Could you check a few things on this model? Use its own coordinates, in mm. Round coordinates to 2 decimals unless told otherwise and drop trailing zeros. Loops run counter-clockwise (first coordinate to the right, second up) from the corner with the lowest first, then second, coordinate; pieces in that order, holes last. Notation, with made-up numbers: M 49.5,-24.5 L 95.5,-24.5 A17 cw 95.5,8.5 Z; hole C 46.5,64 d7. An arc over 180 degrees is marked long. Answer in a Markdown table with one row per item.
```python
from build123d import *

# Parameters (mm, degrees)
ESQUISSE2_W             = 10
ESQUISSE2_H             = 10
BOSS_EXTRU_1_DEPTH      = 90
ESQUISSE3_W             = 10
ESQUISSE3_H             = 150
ESQUISSE3_R             = 2.5
BOSS_EXTRU_2_DEPTH      = 10
ESQUISSE4_R             = 2.5
ENL_V_MAT_EXTRU_1_DEPTH = 10
BOSS_EXTRU_3_DEPTH      = 10


with BuildPart() as part:
    # Esquisse2 → Boss.-Extru.1 (new body)
    with BuildSketch(Plane(origin=(0, 0, 0), x_dir=(0, 0, -1), z_dir=(1, 0, 0))):
        Rectangle(ESQUISSE2_W, ESQUISSE2_H)
    extrude(amount=BOSS_EXTRU_1_DEPTH)

    # Esquisse3 → Boss.-Extru.2 (add)
    with BuildSketch(Plane(origin=(90, 0, 0), x_dir=(0, 0, -1), z_dir=(1, 0, 0))):
        with Locations((0, -70)):
            Rectangle(ESQUISSE3_W, ESQUISSE3_H)
        with Locations((0, -140)):
            Circle(ESQUISSE3_R, mode=Mode.SUBTRACT)
        with Locations((0, -130)):
            Circle(ESQUISSE3_R, mode=Mode.SUBTRACT)
        with Locations((0, -120)):
            Circle(ESQUISSE3_R, mode=Mode.SUBTRACT)
        with Locations((0, -110)):
            Circle(ESQUISSE3_R, mode=Mode.SUBTRACT)
        with Locations((0, -100)):
            Circle(ESQUISSE3_R, mode=Mode.SUBTRACT)
        with Locations((0, -90)):
            Circle(ESQUISSE3_R, mode=Mode.SUBTRACT)
        with Locations((0, -80)):
            Circle(ESQUISSE3_R, mode=Mode.SUBTRACT)
        with Locations((0, -70)):
            Circle(ESQUISSE3_R, mode=Mode.SUBTRACT)
        with Locations((0, -60)):
            Circle(ESQUISSE3_R, mode=Mode.SUBTRACT)
        with Locations((0, -50)):
            Circle(ESQUISSE3_R, mode=Mode.SUBTRACT)
        with Locations((0, -40)):
            Circle(ESQUISSE3_R, mode=Mode.SUBTRACT)
        with Locations((0, -30)):
            Circle(ESQUISSE3_R, mode=Mode.SUBTRACT)
    extrude(amount=BOSS_EXTRU_2_DEPTH)

    # Esquisse4 → Enlèv. mat.-Extru.1 (cut)
    with BuildSketch(Plane(origin=(0, 0, -5), x_dir=(-1, 0, 0), z_dir=(0, 0, -1))):
        with Locations((-5, 0)):
            Circle(ESQUISSE4_R)
        with Locations((-15, 0)):
            Circle(ESQUISSE4_R)
        with Locations((-25, 0)):
            Circle(ESQUISSE4_R)
        with Locations((-35, 0)):
            Circle(ESQUISSE4_R)
        with Locations((-45, 0)):
            Circle(ESQUISSE4_R)
        with Locations((-55, 0)):
            Circle(ESQUISSE4_R)
        with Locations((-65, 0)):
            Circle(ESQUISSE4_R)
        with Locations((-75, 0)):
            Circle(ESQUISSE4_R)
        with Locations((-85, 0)):
            Circle(ESQUISSE4_R)
    extrude(amount=-ENL_V_MAT_EXTRU_1_DEPTH, mode=Mode.SUBTRACT)

    # Esquisse5 → Boss.-Extru.3 (add)
    with BuildSketch(Plane(origin=(0, 0, -5), x_dir=(-1, 0, 0), z_dir=(0, 0, -1))):
        Polygon((-75, -5), (-90, -25), (-90, -5), align=None)
    extrude(amount=-BOSS_EXTRU_3_DEPTH)


solid = part.part
```
1) Will these pins go through, and if not, where does the flat tip stop? P1, Ø3, axis at y = -50.5, z = -2.5, coming from the -X side; P2, Ø1.5, axis at x = 85.5, z = 2.5, coming from the -Y side; P3, Ø6, axis at y = -19.5, z = -4, coming from the -X side (3 decimals).
Computed:
| item | result |
|---|---|
| P1 | stops at x = 90 |
| P2 | stops at y = -20 |
| P3 | stops at x = 83.625 |
2) I want a section at B-B, the plane x = 65. Please give me the cut outline in (y, z).
Computed:
| item | result |
|---|---|
| outline | M -5,-5 L -2.5,-5 L -2.5,5 L -5,5 Z; M 2.5,-5 L 5,-5 L 5,5 L 2.5,5 Z |
3) I need wall thicknesses on line 1 (X direction, y = -101, z = 2.5); line 2 (Y direction, x = 25, z = 3); line 3 (Y direction, x = 37, z = 0.5). Which ranges of each line are inside material? Lowest first, please.
Computed:
| item | result |
|---|---|
| line 1 | x = 90 to 100 |
| line 2 | y = -5 to -2.5, 2.5 to 5 |
| line 3 | y = -5 to -1.5, 1.5 to 5 |
4) I want a section at A-A, the plane y = -100. Please give me the cut outline in (x, z), plus the area to 3 significant figures.
Computed:
| item | result |
|---|---|
| outline | M 90,-5 L 100,-5 L 100,-2.5 L 90,-2.5 Z; M 90,2.5 L 100,2.5 L 100,5 L 90,5 Z |
| area | 50.0 mm² |
5) I want a section at C-C, the plane z = 0. State how many separate pieces and enclosed holes the cut face has, plus the area to 3 significant figures.
Computed:
| item | result |
|---|---|
| separate pieces | 13 |
| enclosed holes | 9 |
| area | 1,770 mm² |
6) If we mould it in two halves opening along Y, with no side actions, what happens to faces 1 (the face through (91, -42, 5)), 2 (the face through (82.395, -14.86, -0.07)), 3 (the face through (94.93, -137.52, 0.33))? For each: released by +Y, released by -Y, zero draft, split by the parting line, or undercut.
Computed:
| item | result |
|---|---|
| face 1 | zero draft |
| face 2 | released by -Y |
| face 3 | undercut |
7) I want a section at D-D, the plane y = -64. Please give me the cut outline in (x, z), plus the area to 3 significant figures.
Computed:
| item | result |
|---|---|
| outline | M 90,-5 L 100,-5 L 100,5 L 90,5 Z |
| area | 100 mm² |
